CAD build for the part. Positions are in the model's coordinates, mm. Face numbers are marked on the shaded views. A direction names the side the tool comes from. Round coordinates to 2 decimals unless told otherwise and drop trailing zeros. Loops run counter-clockwise (first coordinate to the right, second up) from the corner with the lowest first, then second, coordinate; pieces in that order, holes last.
from build123d import *

# Parameters (mm, degrees)
F1_DEPTH = 76.2
F2_W     = 25.4
F2_H     = 25.4
F3_DEPTH = 101.6


with BuildPart() as f1:
    # F0 (on Front) → F1 (new body)
    with BuildSketch(Plane.XZ):
        Polygon((0, 50.8), (0, 0), (127, 0), (127, 25.4), (25.4, 50.8), align=None)
    extrude(amount=F1_DEPTH)

    # F2 (on face) → F3 (cut)
    with BuildSketch(Plane.YZ.offset(127)):
        with Locations((-63.5, 38.1)):
            Rectangle(F2_W, F2_H)
        with Locations((-12.7, 38.1)):
            Rectangle(F2_W, F2_H)
    extrude(amount=-F3_DEPTH, mode=Mode.SUBTRACT)


solid = f1.part
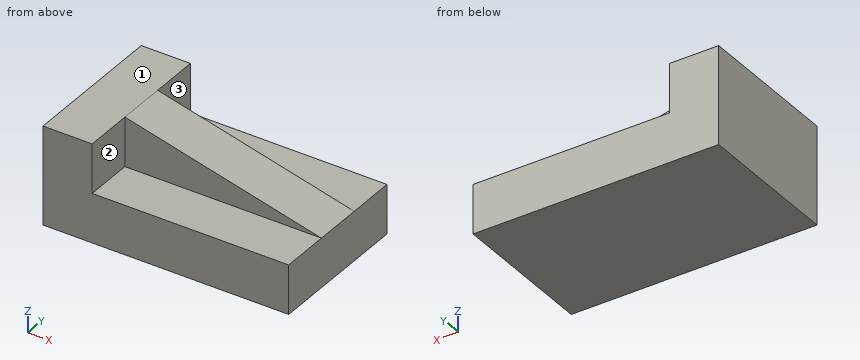
Item 1: Cut at B-B (x = 80). List the corners of the cut face in (y, z), plus the area to 3 significant figures.
Verdict:
outline: (-76.2, 0) - (0, 0) - (0, 25.4) - (-25.4, 25.4) - (-25.4, 37.15) - (-50.8, 37.15) - (-50.8, 25.4) - (-76.2, 25.4) - close
area: 2,230 mm2
Item 2: Cut at A-A (z = 46). List the corners of the cut face in (x, y).
Verdict:
outline: (0, -76.2) - (25.4, -76.2) - (25.4, -50.8) - (44.6, -50.8) - (44.6, -25.4) - (25.4, -25.4) - (25.4, 0) - (0, 0) - close
Item 3: Cut at C-C (y = -63). List the corners of the cut face in (x, z).
Verdict:
outline: (0, 0) - (127, 0) - (127, 25.4) - (25.4, 25.4) - (25.4, 50.8) - (0, 50.8) - close
Item 4: Wall check: L1, parallel to Z at x = 40.5, y = -13; L2, parallel to Y at x = 31, z = 44.5. Give the ranges that are in metal, low to high.
Verdict:
L1: z = 0 to 25.4
L2: y = -50.8 to -25.4
Item 5: Flat gauge pins, fed straight in: P1, Ø12.5, axis at y = -59, z = 42, coming from the +X side; P2, Ø20.5, axis at x = 90.5, z = 44.5, coming from the -Y side; P3, Ø12, axis at x = 52, y = -15.5, coming from the +Z side. Where does each tip first touch, or does it go through?
Verdict:
P1: stops at x = 25.4
P2: stops at y = -50.8
P3: stops at z = 25.4
Item 6: 3-axis set-ups, long thin cutter, end or side, ignore diameter. For the marked faces 1, 2 and 3: which of +Z, -Z, +X, -X, +Y, -Y reach the whole face in a straight line?
Verdict:
face 1: +Z, +X, -X, +Y, -Y
face 2: +Z, +X, -Y
face 3: +Z, +X, +Y
